Autodesk Inventor part; units mm, degrees
ref_plane "YZ Plane" through (0, 0, 0) normal (1, 0, 0) x (0, 1, 0)
ref_plane "XZ Plane" through (0, 0, 0) normal (0, 1, 0) x (-1, 0, 0)
ref_plane "XY Plane" through (0, 0, 0) normal (0, 0, 1) x (1, 0, 0)
sketch "Sketch1" plane through (0, 0, 0) normal (0, 0, 1) x (1, 0, 0)
  line L0 (-10.2, -12.5) -> (0, -12.5)
  line L1 (0, -12.5) -> (0, 12.5)
  line L2 (0, 12.5) -> (-10.2, 12.5)
  line L3 (-10.2, 12.5) -> (-10.2, -12.5)
  point P0 (0, 0)
  dimension "MIRROR_WIDTH" = 10.2
  dimension "WIDTH" = 10.2
  dimension "LENGTH" = 25
  dimension "d3" = 12.5
extrude "Extrusion1" add sketch "Sketch1" along normal blind 6.35
sketch "Sketch2" plane through (0, 0, 6.35) normal (0, 0, 1) x (1, 0, 0)
  line L0 (0, 12.5) -> (2, 12.5)
  line L1 (2, 12.5) -> (2, -12.5)
  line L2 (2, -12.5) -> (0, -12.5)
  line L3 (0, -12.5) -> (0, 12.5)
  point P0 (0, 0)
  dimension "d6" = 2
  dimension "d7" = 25
  dimension "d8" = 12.5
  dimension "d9" = 0
extrude "Extrusion2" [suppressed]
sketch "Sketch3" plane through (0, 0, 6.35) normal (0, 0, 1) x (1, 0, 0)
  point P0 (0, 0)
  point P1 (-5.1, 0)
  dimension "d12" = 5.1
  dimension "d13" = 0
hole "Hole1" at (-5.1, 0, 6.35) direction (0, 0, -1) diameter 4.5 depth 12.3
sketch "Sketch4" plane through (0, 0, 0) normal (0, 0, -1) x (-1, 0, 0)
  circle A0 centre (5.1, 0) radius 2.25
  line L0 (5.1, -5.5455) -> (5.1, -4.4545) construction
  line L1 (6.15, -5.5455) -> (6.15, -4.4545)
  line L2 (4.05, -4.4545) -> (4.05, -5.5455)
  arc A1 (4.05, -5.5455) -> (6.15, -5.5455) centre (5.1, -5.5455) ccw
  arc A2 (6.15, -4.4545) -> (4.05, -4.4545) centre (5.1, -4.4545) ccw
  point P0 (0, 0)
  point P1 (5.1, -5)
  point P2 (5.1, 5)
  dimension "d21" = 0
  dimension "d22" = 0
  dimension "d23" = 5
  dimension "d24" = 5
  dimension "d43" = 1.05
  dimension "d44" = 1.091
hole "Hole2" at (-5.1, 5, 0) direction (0, 0, 1) diameter 2.1 end through all
extrude "Extrusion3" cut sketch "Sketch4" against normal through all contours A1 L2 A2 L1
chamfer "Chamfer1" distance 1 angle 45 4 edges at (-10.2, -12.5, 3.175) (0, -12.5, 3.175) (0, 12.5, 3.175) (-10.2, 12.5, 3.175)
sketch "Sketch6" plane through (0, -11.5, 0) normal (1, 0, 0) x (0, 0, -1)
  circle A0 centre (-18.7, 11.5) radius 12.7
  point P0 (0, 11.5)
  dimension "d50" = 25.4
  dimension "d51" = 0
  dimension "d52" = 18.7
extrude "Extrusion4" cut sketch "Sketch6" against normal up to surface (10.2 mm away)
equation "\"WIDTH\" = MIRROR_WIDTH"
equation "\"d7\" = LENGTH"
properties part number "POLARIS-K05S1-adapter"
Can you work these out from the model? Positions are in its coordinate system, mm. A direction names the side the tool comes from. Give positions to 0.01 mm unless a question says otherwise; leave off trailing zeros. Write each loop counter-clockwise with the first axis right and the second up, starting at its lowest first coordinate (ties: lowest second). Pieces come first, ordered by that corner, then holes. Notation, with made-up numbers: (23, -31) - (48, -31) arc R15 ccw to (48, -21) - close; hole circle Ø5 at (-25, 71). An arc over 180 degrees is marked (long way). Write item = value, one per line. Start each with the question number.
1. On a 3-axis mill with a long thin cutter (end or side, diameter ignored), from which of +Z, -Z, +X, -X, +Y, -Y can I reach the whole of each face in a straight line? I mean faces 1 (the face through (-5.123, -3.405, 3.131)), 2 (the face through (-5, 12.5, 3)). Say none if no direction works.
2. Thinking about a two-plate mould opening in Y: for faces 3 (the face through (0, 0, 3)), 4 (the face through (-9.7, -12, 3.2)), 5 (the face through (-4.05, -5, 3)), which applies, released by +Y, released by -Y, zero draft, split by the parting line, or undercut?
3. Imagine slicing it at C-C (z = 1.5). Please give me the cut outline in (x, y).
4. Please list where these lines run through material, in increasing order: line 1 (Y direction, x = -5.1, z = 2.5); line 2 (X direction, y = 0, z = 4.5); line 3 (Y direction, x = -4.5, z = 5.5).
5. Imagine slicing it at A-A (y = 0). Please give me the cut outline in (x, z), and give its area (3 significant figures).
6. Imagine slicing it at B-B (x = -5.1). Please give me the cut outline in (y, z).
7. For pin 1 (1.2 mm diameter, centred on y = -5, z = 4.5, fed in from +X), with a flat end and sliding along its axis, tell me the tip position at first contact or that it passes through.
8. Imagine slicing it at D-D (y = 5). Please give me the cut outline in (x, z), and give its area (3 significant figures).
Worked answers:
q1.face_1 = +Z, -Z
q1.face_2 = +Z, -Z, +X, -X, +Y
q2.face_3 = zero draft
q2.face_4 = released by -Y
q2.face_5 = undercut
q3.outline = (-10.2, -11.5) - (-9.2, -12.5) - (-1, -12.5) - (0, -11.5) - (0, 11.5) - (-1, 12.5) - (-9.2, 12.5) - (-10.2, 11.5) - close; hole circle Ø4.5 at (-5.1, 0); hole (-6.15, -5.55) arc R1.05 ccw to (-4.05, -5.55) - (-4.05, -4.45) arc R1.05 ccw to (-6.15, -4.45) - close; hole circle Ø2.1 at (-5.1, 5)
q4.line_1 = -12.5 to -6.6, -3.4 to -2.25, 2.25 to 3.95, 6.05 to 12.5
q4.line_2 = -10.2 to -7.35, -2.85 to 0
q4.line_3 = -12.5 to -6.41, -3.59 to -2.17, 2.17 to 4.14, 5.86 to 12.5
q5.outline = (-10.2, 0) - (-7.35, 0) - (-7.35, 6) - (-10.2, 6) - close; (-2.85, 0) - (0, 0) - (0, 6) - (-2.85, 6) - close
q5.area = 34.2 mm2
q6.outline = (-12.5, 0) - (-6.6, 0) - (-6.6, 6.35) - (-12.5, 6.35) - close; (-3.4, 0) - (-2.25, 0) - (-2.25, 6.2) arc R12.7 cw to (-2.96, 6.35) - (-3.4, 6.35) - close; (2.25, 0) - (3.95, 0) - (3.95, 6.35) - (2.96, 6.35) arc R12.7 cw to (2.25, 6.2) - close; (6.05, 0) - (12.5, 0) - (12.5, 6.35) - (6.05, 6.35) - close
q7.pin_1 = 0
q8.outline = (-10.2, 0) - (-6.15, 0) - (-6.15, 6.35) - (-10.2, 6.35) - close; (-4.05, 0) - (0, 0) - (0, 6.35) - (-4.05, 6.35) - close
q8.area = 51.4 mm2
